Could you check a few things on this model? Use its own coordinates, in mm. A direction names the side the tool comes from. Round coordinates to 2 decimals unless told otherwise and drop trailing zeros. Loops run counter-clockwise (first coordinate to the right, second up) from the corner with the lowest first, then second, coordinate; pieces in that order, holes last. Notation, with made-up numbers: (-14, 17) -> (37, 17) arc R15 cw to (37, 28) -> close; hole circle Ø9 at (-4, 45). An arc over 180 degrees is marked (long way). One line per item, written item: value.
```python
from build123d import *

# Parameters (mm, degrees)
F0_R     = 63.5
F1_DEPTH = 101.6
F3_R     = 63.5
F4_DEPTH = 50.8
F5_W     = 108.3593287468
F5_H     = 241.9045526981
F6_DEPTH = 76.2


with BuildPart() as f1:
    # F0 (on Front) → F1 (new body)
    with BuildSketch(Plane.XZ):
        with BuildLine():
            Line((-254, -127), (0, -127))
            ThreePointArc((0, -127), (127, 0), (0, 127))
            Line((0, 127), (-254, 127))
            Line((-254, 127), (-254, -127))
        make_face()
        Circle(F0_R, mode=Mode.SUBTRACT)
    extrude(amount=F1_DEPTH)



with BuildPart() as f4:
    # F3 (on offset) → F4 (new body)
    with BuildSketch(Plane.XZ.offset(177.8)):
        with BuildLine():
            Line((0, 127), (-254, 127))
            Line((-254, 127), (-254, -127))
            Line((-254, -127), (0, -127))
            ThreePointArc((0, -127), (127, 0), (0, 127))
        make_face()
        Circle(F3_R, mode=Mode.SUBTRACT)
    extrude(amount=F4_DEPTH)


with BuildPart() as f1_1:
    add(f1.part)

    add(f4.part)  # F6 merges F4
    # F5 (on face) → F6 (join, through all)
    with BuildSketch(Plane.XZ.offset(101.6)):
        with Locations((-199.8203356266, 6.0477236509)):
            Rectangle(F5_W, F5_H)
    extrude(amount=F6_DEPTH)


solid = f1_1.part
```
(1) Imagine slicing it at B-B on z = 0. Write out the boundary of the cut face in (x, y).
Results below:
outline: (-254, -228.6) -> (-63.5, -228.6) -> (-63.5, -177.8) -> (-145.64, -177.8) -> (-145.64, -101.6) -> (-63.5, -101.6) -> (-63.5, 0) -> (-254, 0) -> close; (63.5, -228.6) -> (127, -228.6) -> (127, -177.8) -> (63.5, -177.8) -> close; (63.5, -101.6) -> (127, -101.6) -> (127, 0) -> (63.5, 0) -> close
(2) On a 3-axis mill with a long thin cutter (end or side, diameter ignored), from which of +Z, -Z, +X, -X, +Y, -Y can I reach the whole of each face in a straight line? I mean faces 1 (the face through (-145.641, -139, 4)), 2 (the face through (-129, -203, -127)). Say none if no direction works.
Results below:
face 1: +Z, -Z, +X
face 2: -Z, +X, -X, +Y, -Y
(3) Imagine slicing it at A-A on x = -96. Write out the boundary of the cut face in (y, z).
Results below:
outline: (-228.6, -127) -> (-177.8, -127) -> (-177.8, 127) -> (-228.6, 127) -> close; (-101.6, -127) -> (0, -127) -> (0, 127) -> (-101.6, 127) -> close
(4) We'd pull the mould along Z, two halves only. Please class faces 3 (the face through (-201, -139, -114.905)), 4 (the face through (-13.77, -202.84, -61.99)), 5 (the face through (-254, -113, -2)): +Z half, -Z half, draft (parallel to the pull), parting line (faces both ways), or undercut.
Results below:
face 3: -Z half
face 4: undercut
face 5: draft
(5) For pin 1 Ø23 at (y, z) = (-150.5, -8) entering from +X; pin 2 Ø23 at (x, y) = (-197, -126.5) entering from -Z, each with a flat end and sliding along its axis, tell me the tip position at first contact or that it passes through.
Results below:
pin 1: stops at x = -145.64
pin 2: stops at z = -114.9
(6) Imagine slicing it at C-C on y = -59. Write out the boundary of the cut face in (x, z), then the cut area to 3 significant figures.
Results below:
outline: (-254, -127) -> (0, -127) arc R127 ccw to (0, 127) -> (-254, 127) -> close; hole circle Ø127 at (0, 0)
area: 77,200 mm²
(7) Imagine slicing it at D-D on y = -166. Write out the boundary of the cut face in (x, z).
Results below:
outline: (-254, -114.9) -> (-145.64, -114.9) -> (-145.64, 127) -> (-254, 127) -> close
(8) Please list where these lines run through material, in increasing order: L1, parallel to Y at x = 77, z = 35.5; L2, parallel to X at y = -142, z = -34.5; L3, parallel to X at y = -71.5, z = 11.
Results below:
L1: y = -228.6 to -177.8, -101.6 to 0
L2: x = -254 to -145.64
L3: x = -254 to -62.54, 62.54 to 126.52
